Could you check a few things on this model? Use its own coordinates, in mm. Coordinates: 2 decimals unless noted, no trailing zeros. Loops run counter-clockwise (first coordinate to the right, second up) from the corner with the lowest first, then second, coordinate; pieces in that order, holes last. Notation, with made-up numbers: M 73,70.5 L 126,70.5 A13 ccw 126,84.5 Z; hole C 48,41.5 d1. An arc over 180 degrees is marked long. Write each question's results on one line, items separated by ' | '.
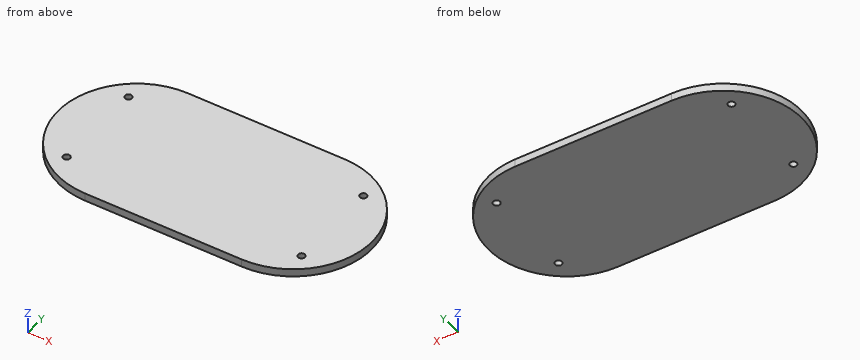
```python
from build123d import *

# Parameters (mm, degrees)
F0_W     = 100
F0_H     = 100
F1_DEPTH = 5
F3_D     = 4.4


with BuildPart() as f1:
    # F0 (on Top) → F1 (new body)
    with BuildSketch(Plane.XY):
        Rectangle(F0_W, F0_H)
        with BuildLine():
            ThreePointArc((50, -50), (100, 0), (50, 50))
            Line((50, 50), (50, -50))
        make_face()
        with BuildLine():
            Line((-50, -50), (-50, 50))
            ThreePointArc((-50, 50), (-100, 0), (-50, -50))
        make_face()
    extrude(amount=F1_DEPTH)

    # F3 (through all)
    with Locations(Plane.XY.offset(5)):
        with Locations((-75, 30), (75, 30), (75, -30), (-75, -30)):
            Hole(F3_D / 2)


solid = f1.part
```
(1) Imagine slicing it at B-B, the plane x = 75. List the corners of the cut face in (y, z) for me.
Reported:
outline: M -43.3,0 L -32.2,0 L -32.2,5 L -43.3,5 Z; M -27.8,0 L 27.8,0 L 27.8,5 L -27.8,5 Z; M 32.2,0 L 43.3,0 L 43.3,5 L 32.2,5 Z
(2) Imagine slicing it at D-D, the plane y = -15.5. List the corners of the cut face in (x, z) for me, and give its area (3 significant figures).
Reported:
outline: M -97.54,0 L 97.54,0 L 97.54,5 L -97.54,5 Z | area: 975 mm2
(3) Imagine slicing it at C-C, the plane y = 20.5. List the corners of the cut face in (x, z) for me.
Reported:
outline: M -95.6,0 L 95.6,0 L 95.6,5 L -95.6,5 Z
(4) Imagine slicing it at A-A, the plane z = 2.6. List the corners of the cut face in (x, y) for me.
Reported:
outline: M -50,-50 L 50,-50 A50 ccw 50,50 L -50,50 A50 ccw Z; hole C -75,-30 d4.4; hole C -75,30 d4.4; hole C 75,-30 d4.4; hole C 75,30 d4.4
(5) Please list where these lines run through material, in increasing order: probe 1 along Y at (x, z) = (75, 3.9); probe 2 along Y at (x, z) = (73, 0.45); probe 3 along X at (y, z) = (31, 2.05). Write a range as from..to.
Reported:
probe 1: y = -43.3..-32.2, -27.8..27.8, 32.2..43.3 | probe 2: y = -44.4..-30.92, -29.08..29.08, 30.92..44.4 | probe 3: x = -89.23..-76.96, -73.04..73.04, 76.96..89.23
